CAD build for the part. Positions are in the model's coordinates, mm. A direction names the side the tool comes from. Give positions to 0.01 mm unless a question says otherwise; leave off trailing zeros. Order: outer loops, then holes, each group sorted by start corner. A loop starts at its lowest first (then second) coordinate and runs counter-clockwise, first axis right, second up.
```python
from build123d import *

# Parameters (mm, degrees)
SKETCH1_W           = 30
SKETCH1_H           = 26
SKETCH1_W_2         = 16.187399031
SKETCH1_H_2         = 14.6365105
BOSS_EXTRUDE1_DEPTH = 1.8
SKETCH1_3_W         = 16.187399031
SKETCH1_3_H         = 14.6365105
BOSS_EXTRUDE2_DEPTH = 8
SKETCH2_W           = 4.688292782
SKETCH2_H           = 3.45561668
SKETCH2_H_2         = 3.896759234
BOSS_EXTRUDE3_DEPTH = 0.5


with BuildPart() as part:
    # Sketch1 → Boss-Extrude1 (new body)
    # profile 1 of 2: a face of its own
    with BuildSketch(Plane(origin=(0, 0, 0), x_dir=(1, 0, 0), z_dir=(0, 1, 0))):
        with Locations((15, 13)):
            Rectangle(SKETCH1_W, SKETCH1_H)
        with Locations((21.227786753, 8.239095315)):
            Rectangle(SKETCH1_W_2, SKETCH1_H_2, mode=Mode.SUBTRACT)
    # profile 2 of 2: a face of its own
    with BuildSketch(Plane(origin=(0, 0, 0), x_dir=(1, 0, 0), z_dir=(0, 1, 0))):
        with Locations((21.227786753, 8.239095315)):
            Rectangle(SKETCH1_W_2, SKETCH1_H_2)
    extrude(amount=BOSS_EXTRUDE1_DEPTH)

    # Sketch1_3 → Boss-Extrude2 (add)
    with BuildSketch(Plane(origin=(0, 0, 0), x_dir=(1, 0, 0), z_dir=(0, 1, 0))):
        with Locations((21.227786753, 8.239095315)):
            Rectangle(SKETCH1_3_W, SKETCH1_3_H)
    extrude(amount=BOSS_EXTRUDE2_DEPTH)

    # Sketch2 → Boss-Extrude3 (add)
    with BuildSketch(Plane(origin=(0, 1.8, 0), x_dir=(1, 0, 0), z_dir=(0, 1, 0))):
        with Locations((2.344146391, 22.502945868)):
            Rectangle(SKETCH2_W, SKETCH2_H)
        with Locations((2.344146391, 12.540476505)):
            Rectangle(SKETCH2_W, SKETCH2_H_2)
        with Locations((2.344146391, 4.048482326)):
            Rectangle(SKETCH2_W, SKETCH2_H_2)
    extrude(amount=BOSS_EXTRUDE3_DEPTH)


solid = part.part
```
Item 1: Slice it at A-A (z = -9.75). Give the cut face in (x, y), and give its area (3 significant figures).
Item 2: Slice it at B-B (x = 2.75). Give the cut face in (y, z).
Item 3: Tool access for faces 1 (the face through (2, 2.3, -13)), 2 (the face through (21, 5, -0.921)), 3 (the face through (29.321, 5, -8)), 4 (the face through (15, 1, -26)), 5 (the face through (21, 5, -15.557)): list every direction of +Z, -Z, +X, -X, +Y, -Y with a clear straight run to the whole face (end or side of a thin tool).
Item 4: Drop flat-ended pins along their axis: pin 1 Ø1.7 at (x, z) = (2, -22.5) entering from +Y; pin 2 Ø1 at (y, z) = (4.5, -4.5) entering from +X; pin 3 Ø3 at (x, y) = (20, 6.5) entering from +Z. Give the stop position or say it passes through.
Item 5: Wall check: L1, parallel to X at y = 5.5, z = -7; L2, parallel to Z at x = 24.75, y = 6.75; L3, parallel to Y at x = 6.5, z = -8. Give the ranges that are in metal, low to high.
Item 6: Slice it at C-C (y = 6). Give the cut face in (x, z).
Item 7: Slice it at D-D (z = -23). Give the cut face in (x, y), and give its area (3 significant figures).
A:
1. outline: (0, 0) - (30, 0) - (30, 1.8) - (29.32, 1.8) - (29.32, 8) - (13.13, 8) - (13.13, 1.8) - (0, 1.8) - close
1. area: 154 mm2
2. outline: (0, -26) - (1.8, -26) - (1.8, -24.23) - (2.3, -24.23) - (2.3, -20.78) - (1.8, -20.78) - (1.8, -14.49) - (2.3, -14.49) - (2.3, -10.59) - (1.8, -10.59) - (1.8, -6) - (2.3, -6) - (2.3, -2.1) - (1.8, -2.1) - (1.8, 0) - (0, 0) - close
3. face 1: +Z, -Z, -X, +Y
3. face 2: +Z, +X, -X, +Y
3. face 3: +Z, -Z, +X, +Y
3. face 4: -Z, +X, -X, +Y, -Y
3. face 5: -Z, +X, -X, +Y
4. pin 1: stops at y = 2.3
4. pin 2: stops at x = 29.32
4. pin 3: stops at z = -0.92
5. L1: x = 13.13 to 29.32
5. L2: z = -15.56 to -0.92
5. L3: y = 0 to 1.8
6. outline: (13.13, -15.56) - (29.32, -15.56) - (29.32, -0.92) - (13.13, -0.92) - close
7. outline: (0, 0) - (30, 0) - (30, 1.8) - (4.69, 1.8) - (4.69, 2.3) - (0, 2.3) - close
7. area: 56.3 mm2
